Model file for the job. Use its own axes, mm. A direction names the side the tool comes from. Give positions to 0.01 mm unless a question says otherwise; leave off trailing zeros. Loops run counter-clockwise (first coordinate to the right, second up) from the corner with the lowest first, then second, coordinate; pieces in that order, holes last. Notation, with made-up numbers: (-30.75, -29.75) -> (18.25, -29.75) arc R30 cw to (18.25, 3.25) -> close; hole circle Ø4 at (31.5, 39). An arc over 180 degrees is marked (long way). Use CSV: the item, a comma, the result in double quotes. Start each with the question number.
(1) 3-axis set-ups, long thin cutter, end or side, ignore diameter. For faces 5 (the flat face through (-1, 11, -3.25)), 6 (the flat face through (27.5, 0, 0)): which of +Z, -Z, +X, -X, +Y, -Y reach the whole face in a straight line?
(2) Cut at B-B on y = 0. Write the cut outline in (x, z).
(3) Cut at A-A on x = -25. Write the cut outline in (y, z).
(4) Drill centre lines: probe 1 along Y at (x, z) = (25, 0.5); probe 2 along Y at (x, z) = (0, 2); probe 3 along X at (y, z) = (-9, 1.25). Where is each one in solid material? Low to high.
(5) Flat gauge pin, fed straight in: pin 1 (4.5 mm diameter, centred on x = -25, y = -4.98, fed in from +Z). Where does the tip first touch, or does it go through?
(6) Cut at C-C on x = -16. Write the cut outline in (y, z).
(7) Pull direction Y, two halves, no side cores. Call faces 1 (the flat face through (0, -9.983, 0)), 2 (the flat face through (1, -15.6, 0)), 3 (the flat face through (-41.6, 0, 0)), 4 (the flat face through (20, 5, 0)): pulls with the +Y half, pulls with the -Y half, needs draft (parallel to the pull), parting line crosses it, or undercut.
(8) Cut at D-D on z = -2.5. Write the cut outline in (x, y), then the cut area to 3 significant figures.
Autodesk Inventor part; units mm, degrees
ref_plane "YZ Plane" through (0, 0, 0) normal (1, 0, 0) x (0, 1, 0)
ref_plane "XZ Plane" through (0, 0, 0) normal (0, 1, 0) x (-1, 0, 0)
ref_plane "XY Plane" through (0, 0, 0) normal (0, 0, 1) x (1, 0, 0)
sketch "Sketch1" plane through (0, 0, 0) normal (0, 0, 1) x (1, 0, 0)
  line L0 (-20, 10.0166) -> (20, 10.0166)
  line L1 (19.9334, -9.9833) -> (-19.9334, -9.9833)
  line L2 (-20, 10.0166) -> (19.9334, -9.9833) construction
  line L3 (20, 10.0166) -> (-19.9334, -9.9833) construction
  line L4 (-41.6, 15.6) -> (41.6, 15.6)
  line L5 (41.6, 15.6) -> (41.6, -15.6)
  line L6 (41.6, -15.6) -> (-41.6, -15.6)
  line L7 (-41.6, -15.6) -> (-41.6, 15.6)
  line L8 (-41.6, 15.6) -> (41.6, -15.6) construction
  line L9 (41.6, 15.6) -> (-41.6, -15.6) construction
  line L10 (-20, 1.0167) -> (-27.5, 1.0167)
  line L11 (-27.5, 1.0167) -> (-27.5, -0.9833)
  line L12 (-27.5, -0.9833) -> (-19.9334, -0.9833)
  line L13 (20, 1.0167) -> (27.5, 1.0167)
  line L14 (27.5, 1.0167) -> (27.5, -0.9833)
  line L15 (27.5, -0.9833) -> (19.9334, -0.9833)
  line L16 (-20, 1.0167) -> (-20, 10.0166)
  line L17 (-19.9334, -9.9833) -> (-19.9334, -0.9833)
  line L18 (19.9334, -0.9833) -> (19.9334, -9.9833)
  line L19 (20, 1.0167) -> (20, 10.0166)
  point P0 (0, 0)
  point P1 (-27.5, 0.0167)
  point P2 (-0.0333, 0.0167)
  point P3 (0, 10.0166)
  point P4 (0, 0)
  dimension "CInt" = 40
  dimension "LInt" = 20
  dimension "Cext" = 83.2
  dimension "Lext" = 31.2
  dimension "Cpeq" = 7.5
  dimension "Lpeq" = 2
  dimension "d10" = 7.5
  dimension "d11" = 2
extrude "Extrusion1" add sketch "Sketch1" along normal mid plane 6.5
sketch "Sketch8" plane through (0, 0, 3.25) normal (0, 0, 1) x (1, 0, 0)
  point P0 (0, 0)
hole "Hole1" at (-25, 5.0167, 3.25) direction (0, 0, -1) diameter 5 end through all
pattern_linear "Rectangular Pattern1" count 2 spacing 10 along (0, -1, 0) of "Hole1"
hole "Hole2" at (25, 5.0167, 3.25) direction (0, 0, -1) diameter 5 end through all
pattern_linear "Rectangular Pattern2" count 2 spacing 10 along (0, -1, 0) of "Hole2"
properties part number "Cou-Bon"
Check result:
1,face 5,"-Z, +X, -X, +Y, -Y"
1,face 6,"+Z, -Z"
2,outline,"(-41.6, -3.25) -> (-27.5, -3.25) -> (-27.5, 3.25) -> (-41.6, 3.25) -> close; (27.5, -3.25) -> (41.6, -3.25) -> (41.6, 3.25) -> (27.5, 3.25) -> close"
3,outline,"(-15.6, -3.25) -> (-7.48, -3.25) -> (-7.48, 3.25) -> (-15.6, 3.25) -> close; (-2.48, -3.25) -> (-0.98, -3.25) -> (-0.98, 3.25) -> (-2.48, 3.25) -> close; (1.02, -3.25) -> (2.52, -3.25) -> (2.52, 3.25) -> (1.02, 3.25) -> close; (7.52, -3.25) -> (15.6, -3.25) -> (15.6, 3.25) -> (7.52, 3.25) -> close"
4,probe 1,"-15.6 to -7.48, -2.48 to -0.98, 1.02 to 2.52, 7.52 to 15.6"
4,probe 2,"-15.6 to -9.98, 10.02 to 15.6"
4,probe 3,"-41.6 to -19.93, 19.93 to 41.6"
5,pin 1,"through"
6,outline,"(-15.6, -3.25) -> (-9.98, -3.25) -> (-9.98, 3.25) -> (-15.6, 3.25) -> close; (10.02, -3.25) -> (15.6, -3.25) -> (15.6, 3.25) -> (10.02, 3.25) -> close"
7,face 1,"undercut"
7,face 2,"pulls with the -Y half"
7,face 3,"needs draft"
7,face 4,"undercut"
8,outline,"(-41.6, -15.6) -> (41.6, -15.6) -> (41.6, 15.6) -> (-41.6, 15.6) -> close; hole circle Ø5 at (-25, -4.98); hole (-27.5, -0.98) -> (-19.93, -0.98) -> (-19.93, -9.98) -> (19.93, -9.98) -> (19.93, -0.98) -> (27.5, -0.98) -> (27.5, 1.02) -> (20, 1.02) -> (20, 10.02) -> (-20, 10.02) -> (-20, 1.02) -> (-27.5, 1.02) -> close; hole circle Ø5 at (-25, 5.02); hole circle Ø5 at (25, -4.98); hole circle Ø5 at (25, 5.02)"
8,area,"1,690 mm²"
